Here's how the part is built. I have some questions about the finished solid (model axes, mm). Face numbers are marked on the shaded views. A direction names the side the tool comes from. Round coordinates to 2 decimals unless told otherwise and drop trailing zeros. Write each loop counter-clockwise with the first axis right and the second up, starting at its lowest first coordinate (ties: lowest second). Pieces come first, ordered by that corner, then holes. Notation, with made-up numbers: (-37, -35.5) - (-16, -35.5) arc R24 cw to (-16, -21.5) - close; hole circle Ø2 at (-26.5, 16). An arc over 180 degrees is marked (long way). One line per item, written item: value. Start each with the question number.
Item 1: Imagine slicing it at B-B, the plane x = 4.92. Please give me the cut outline in (y, z).
Item 2: For P1, Ø1.2, axis at x = 4.92, z = 0, coming from the -Y side; P2, Ø2, axis at y = -4.5, z = -2.5, coming from the +X side, each with a flat end and sliding along its axis, tell me the tip position at first contact or that it passes through.
Item 3: Imagine slicing it at A-A, the plane z = 0. Please give me the cut outline in (x, y) (1 decimal).
Item 4: For the marked faces 1 and 2, which set-ups out of +Z, -Z, +X, -X, +Y, -Y let a thin tool reach every point of the face, with its end or its side?
Item 5: Imagine slicing it at C-C, the plane y = 1.5. Please give me the cut outline in (x, z) (3 decimals).
Item 6: Thinking about a two-plate mould opening in Y: for the marked faces 3, 4 and 5, which applies, released by +Y, released by -Y, zero draft, split by the parting line, or undercut?
Item 7: If I drill on line 1 (Y direction, x = 1.3, z = 0) (3 decimals); line 2 (X direction, y = 7.05, z = 0); line 3 (Z direction, x = 10, y = 6.95), over which ranges is the centre line in solid material (lowest first)?
Item 8: Imagine slicing it at D-D, the plane z = 2.05. Please give me the cut outline in (x, y).
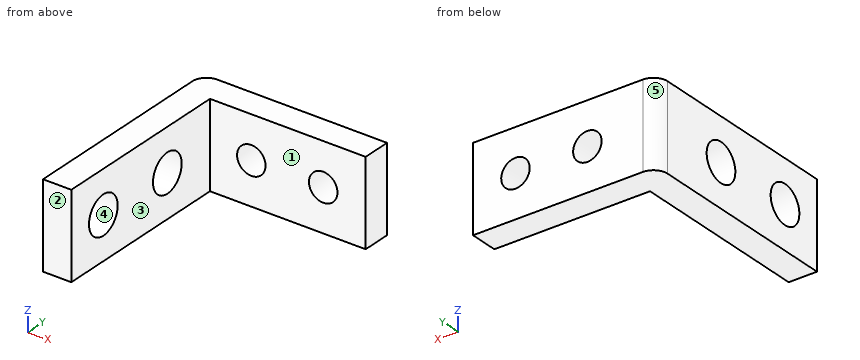
Autodesk Inventor part; units mm, degrees
ref_plane "YZ Plane" through (0, 0, 0) normal (1, 0, 0) x (0, 1, 0)
ref_plane "XZ Plane" through (0, 0, 0) normal (0, 1, 0) x (-1, 0, 0)
ref_plane "XY Plane" through (0, 0, 0) normal (0, 0, 1) x (1, 0, 0)
sketch "Sketch1" plane through (0, 0, 0) normal (1, 0, 0) x (0, 1, 0)
  line L0 (-7.5, 3) -> (7.5, 3)
  line L1 (7.5, 3) -> (7.5, -3)
  line L2 (7.5, -3) -> (-7.5, -3)
  line L3 (-7.5, -3) -> (-7.5, 3)
  line L4 (-7.5, 3) -> (7.5, -3) construction
  line L5 (7.5, 3) -> (-7.5, -3) construction
  point P0 (0, 0)
  dimension "d0" = 15
  dimension "d1" = 6
extrude "Extrusion1" add sketch "Sketch1" along normal blind 2
sketch "Sketch2" plane through (2, 0, 0) normal (1, 0, 0) x (0, 0, -1)
  line L0 (3, 7.5) -> (-3, 7.5)
  line L1 (3, -7.5) -> (3, 7.5)
  line L2 (-3, 7.5) -> (3, 7.5)
  line L3 (3, 7.5) -> (3, 5.5)
  line L4 (3, 5.5) -> (-3, 5.5)
  line L5 (-3, 5.5) -> (-3, 7.5)
  point P0 (0, 0)
  dimension "d4" = 2
extrude "Extrusion2" add sketch "Sketch2" along normal blind 11
fillet "Fillet1" radius 1 1 edges at (0, 7.5, 0)
sketch "Sketch3" plane through (13, 7.5, 3) normal (0, 1, 0) x (1, 0, 0)
  line L0 (0, 6) -> (0, 0) construction
  line L1 (0, 3) -> (-12, 3) construction
  line L2 (-12, 0) -> (-12, 6) construction
  point P0 (-13, 3)
  point P1 (-8.08, 3)
  point P2 (-3, 3)
  dimension "d8" = 5.08
  dimension "d9" = 3
hole "Hole1" at (4.92, 7.5, 0) at (10, 7.5, 0) direction (0, -1, 0) diameter 2.013 end through all
sketch "Sketch4" plane through (2, 0, 0) normal (1, 0, 0) x (0, 0, -1)
  line L0 (-3, -7.5) -> (3, -7.5) construction
  line L1 (0, -7.5) -> (0, 5.5) construction
  line L2 (-3, 5.5) -> (3, 5.5) construction
  line L3 (3, 7.5) -> (-3, 7.5) construction
  point P0 (0, 0)
  point P1 (0, 1.5)
  point P2 (0, -4.5)
  dimension "d17" = 6
  dimension "d18" = 6
hole "Hole2" at (2, 1.5, 0) at (2, -4.5, 0) direction (-1, 0, 0) diameter 2.69 end through all
properties part number "bracket"
Values follow:
1. outline: (5.5, -3) - (7.5, -3) - (7.5, -1.01) - (5.5, -1.01) - close; (5.5, 1.01) - (7.5, 1.01) - (7.5, 3) - (5.5, 3) - close
2. P1: passes through
2. P2: stops at x = 2
3. outline: (0, -7.5) - (2, -7.5) - (2, -5.8) - (0, -5.8) - close; (0, -3.2) - (2, -3.2) - (2, 0.2) - (0, 0.2) - close; (0, 2.8) - (2, 2.8) - (2, 5.5) - (3.9, 5.5) - (3.9, 7.5) - (1, 7.5) arc R1 ccw to (0, 6.5) - close; (5.9, 5.5) - (9, 5.5) - (9, 7.5) - (5.9, 7.5) - close; (11, 5.5) - (13, 5.5) - (13, 7.5) - (11, 7.5) - close
4. face 1: +Z, -Z, +X, -Y
4. face 2: +Z, -Z, +X, -X, -Y
5. outline: (0, -3) - (2, -3) - (2, -1.345) - (0, -1.345) - close; (0, 1.345) - (2, 1.345) - (2, 3) - (0, 3) - close
6. face 3: zero draft
6. face 4: undercut
6. face 5: released by +Y
7. line 1: y = -7.5 to -5.845, -3.155 to 0.155, 2.845 to 7.5
7. line 2: x = 0.16 to 3.91, 5.93 to 8.99, 11.01 to 13
7. line 3: z = -3 to -1.01, 1.01 to 3
8. outline: (0, -7.5) - (2, -7.5) - (2, 5.5) - (13, 5.5) - (13, 7.5) - (1, 7.5) arc R1 ccw to (0, 6.5) - close
